Verification items for this drawing (mm, ordinates from the low corner). Give positions to 0.01 mm unless a question says otherwise; leave off trailing zeros. Write each loop counter-clockwise with the first axis right and the second up, starting at its lowest first coordinate (ties: lowest second). Pieces come first, ordered by that corner, then holes. Notation, with made-up numbers: M 63,25.25 L 102,25.25 A21 ccw 102,53.25 Z; hole C 65,38.25 d7. An arc over 180 degrees is marked long. Use one line per item in the form item = value. Start each with the question number.
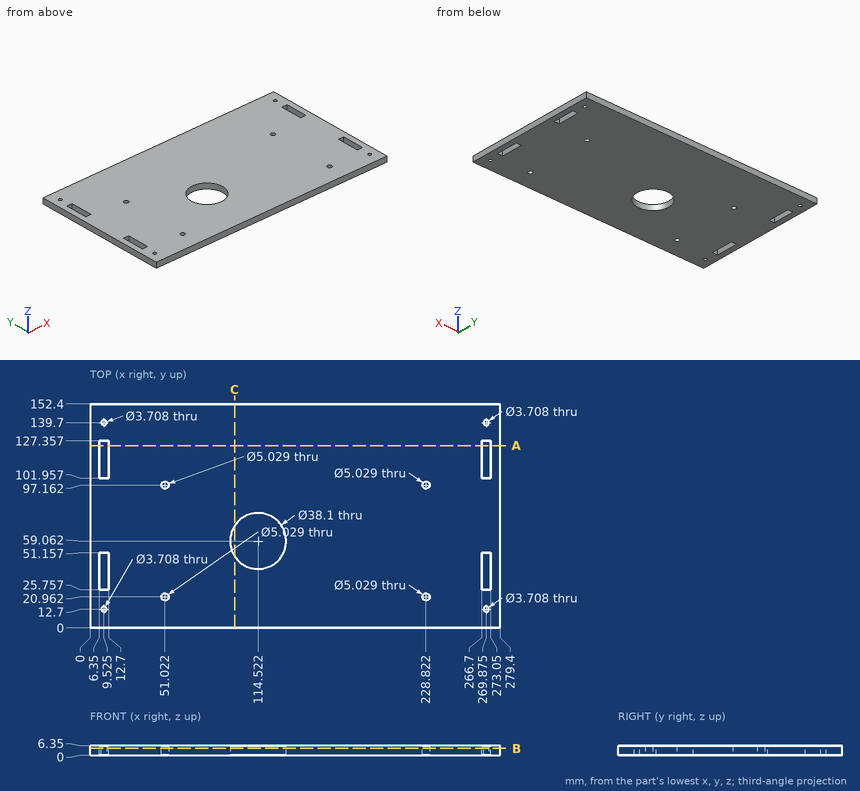
(1) Sectioned sample at C-C, the plane x = 98.5. Record the boundary of the cut face in (y, z).
(2) Sectioned sample at B-B, the plane z = 4.5. State how many separate pieces and enclosed holes the cut face has, plus the area to 3 significant figures.
(3) Sectioned sample at A-A, the plane y = 124. Record the boundary of the cut face in (x, z).
(4) Depth check by flat-ended pin: pin 1 (3 mm diameter, centred on y = 37.5, z = 4.5, fed in from -X); pin 2 (3.5 mm diameter, centred on x = 269.875, y = 139.7, fed in from -Z). Enter the tip coordinate at first touch or a pass-through.
(5) Thickness scan on probe 1 along X at (y, z) = (139.7, 1.75); probe 2 along X at (y, z) = (29, 1.5); probe 3 along X at (y, z) = (47.5, 5.75). Record the ranges inside material, lowest first. Write a range as [from, to].
Numbers:
q1.outline = M 0,0 L 48.76,0 L 48.76,6.35 L 0,6.35 Z; M 69.37,0 L 152.4,0 L 152.4,6.35 L 69.37,6.35 Z
q2.separate_pieces = 1
q2.enclosed_holes = 13
q2.area = 40,700 mm2
q3.outline = M 0,0 L 6.35,0 L 6.35,6.35 L 0,6.35 Z; M 12.7,0 L 266.7,0 L 266.7,6.35 L 12.7,6.35 Z; M 273.05,0 L 279.4,0 L 279.4,6.35 L 273.05,6.35 Z
q4.pin_1 = 0
q4.pin_2 = through
q5.probe_1 = [0, 7.67], [11.38, 268.02], [271.73, 279.4]
q5.probe_2 = [0, 6.35], [12.7, 266.7], [273.05, 279.4]
q5.probe_3 = [0, 6.35], [12.7, 99.38], [129.66, 266.7], [273.05, 279.4]
